from build123d import *

# Parameters (mm, degrees)
EXTRUDE_1_DEPTH      = 4
EXTRUDE_1_DEPTH_BACK = 0.4
SKETCH_1_R           = 4
SKETCH_1_3_R         = 4.175
SKETCH_1_3_R_2       = 4
CUT_EXTRUDE_1_DEPTH  = 3.6
CHAMFER_1_SIZE       = 0.2
FILLET_1_R           = 10


with BuildPart() as part:
    # 草图1 → 凸台-拉伸1 (new, two sides: drawn at the far end of the back side and taken through both)
    with BuildSketch(Plane.XY.offset(-EXTRUDE_1_DEPTH_BACK)):
        with BuildLine():
            ThreePointArc((5.196152423, 3), (-6, 0), (5.196152423, -3))
            Line((5.196152423, -3), (40.803847577, -3))
            ThreePointArc((40.803847577, -3), (52, 0), (40.803847577, 3))
            Line((40.803847577, 3), (5.196152423, 3))
        make_face()
        Circle(SKETCH_1_R, mode=Mode.SUBTRACT)
        with Locations((46, 0)):
            Circle(SKETCH_1_R, mode=Mode.SUBTRACT)
    extrude(amount=EXTRUDE_1_DEPTH + EXTRUDE_1_DEPTH_BACK)

    # 草图1<3> → 切除-拉伸1 (cut)
    # profile 1 of 2: a face of its own
    with BuildSketch(Plane.XY):
        Circle(SKETCH_1_3_R)
        Circle(SKETCH_1_3_R_2, mode=Mode.SUBTRACT)
    # profile 2 of 2: a face of its own
    with BuildSketch(Plane.XY):
        with Locations((46, 0)):
            Circle(SKETCH_1_3_R)
        with Locations((46, 0)):
            Circle(SKETCH_1_3_R_2, mode=Mode.SUBTRACT)
    extrude(amount=CUT_EXTRUDE_1_DEPTH, mode=Mode.SUBTRACT)

    # 倒角1
    # the kernel refuses this chamfer: 0.2 mm, written as the material it takes off along each edge
    with BuildSketch(Plane(origin=(0, 0, 3.6), x_dir=(1, 0, 0), z_dir=(0, -1, 0))) as chamfer_1_piece_1_section:
        Polygon((4, CHAMFER_1_SIZE), (4 + CHAMFER_1_SIZE, 0), (4, 0), align=None)
    chamfer_1_piece_1 = revolve(axis=Axis((0, 0, 3.6), (0, 0, 1)), mode=Mode.PRIVATE)
    chamfer_1_piece_1 = chamfer_1_piece_1 & Plane(origin=(0, 0, 3.709543273), x_dir=(1, 0, 0), z_dir=(0, 0, -1)) * Cylinder(4.175, 17, mode=Mode.PRIVATE)
    add(chamfer_1_piece_1, mode=Mode.SUBTRACT)
    with BuildSketch(Plane(origin=(46, 0, 3.6), x_dir=(1, 0, 0), z_dir=(0, -1, 0))) as chamfer_1_piece_2_section:
        Polygon((4, CHAMFER_1_SIZE), (4 + CHAMFER_1_SIZE, 0), (4, 0), align=None)
    chamfer_1_piece_2 = revolve(axis=Axis((46, 0, 3.6), (0, 0, 1)), mode=Mode.PRIVATE)
    chamfer_1_piece_2 = chamfer_1_piece_2 & Plane(origin=(46, 0, 3.709543273), x_dir=(1, 0, 0), z_dir=(0, 0, -1)) * Cylinder(4.175, 17, mode=Mode.PRIVATE)
    add(chamfer_1_piece_2, mode=Mode.SUBTRACT)
    with BuildSketch(Plane(origin=(46, 0, 0), x_dir=(1, 0, 0), z_dir=(0, -1, 0))) as chamfer_1_piece_3_section:
        Polygon((4, -CHAMFER_1_SIZE), (4 + CHAMFER_1_SIZE, 0), (4, 0), align=None)
    chamfer_1_piece_3 = revolve(axis=Axis((46, 0, 0), (0, 0, 1)), mode=Mode.PRIVATE)
    chamfer_1_piece_3 = chamfer_1_piece_3 & Plane(origin=(46, 0, -0.109543273), x_dir=(1, 0, 0), z_dir=(0, 0, -1)) * Cylinder(4.175, 17, mode=Mode.PRIVATE)
    add(chamfer_1_piece_3, mode=Mode.SUBTRACT)
    with BuildSketch(Plane(origin=(0, 0, 0), x_dir=(1, 0, 0), z_dir=(0, -1, 0))) as chamfer_1_piece_4_section:
        Polygon((4, -CHAMFER_1_SIZE), (4 + CHAMFER_1_SIZE, 0), (4, 0), align=None)
    chamfer_1_piece_4 = revolve(axis=Axis((0, 0, 0), (0, 0, 1)), mode=Mode.PRIVATE)
    chamfer_1_piece_4 = chamfer_1_piece_4 & Plane(origin=(0, 0, -0.109543273), x_dir=(1, 0, 0), z_dir=(0, 0, -1)) * Cylinder(4.175, 17, mode=Mode.PRIVATE)
    add(chamfer_1_piece_4, mode=Mode.SUBTRACT)

    # 圆角1
    fillet_1_edges = [part.edges().sort_by_distance(p)[0] for p in [
        (5.196152423, -3, 1.8),
        (5.196152423, 3, 1.8),
        (40.803847577, 3, 1.8),
        (40.803847577, -3, 1.8),
    ]]
    fillet(fillet_1_edges, radius=FILLET_1_R)


solid = part.part
Design review of the part built by this model. Coordinates are the model's own, in mm. A direction names the side the tool comes from. Coordinates: 2 decimals unless noted, no trailing zeros. Write each loop counter-clockwise with the first axis right and the second up, starting at its lowest first coordinate (ties: lowest second). Pieces come first, ordered by that corner, then holes. Notation, with made-up numbers: (9.25, -32) - (67.25, -32) arc R10 ccw to (67.25, -13) - close; hole circle Ø11 at (25.25, -33). An arc over 180 degrees is marked (long way). Use one line per item in the form item = value.
Q1. Insertion check: pin 1 Ø6.5 at (x, y) = (0, 0) entering from -Z; pin 2 Ø2 at (y, z) = (4.5, 2) entering from -X; pin 3 Ø1.3 at (x, z) = (17, 1.5) entering from +Y; pin 4 Ø1.5 at (y, z) = (-4, 1.5) entering from -X. Each pin has a flat end and moves straight along its axis. Give the tip position at first contact, or say it passes through.
Taken from the geometry:
pin_1 = through
pin_2 = -4.87
pin_3 = 3
pin_4 = -5.04
Q2. Consider section A-A (x = 46). Write out the cut boundary in (y, z) (3 decimals), plus the area to 3 significant figures.
Taken from the geometry:
outline = (-6, -0.4) - (-4, -0.4) - (-4, -0.2) - (-4.175, -0.025) - (-4.175, 3.625) - (-4, 3.8) - (-4, 4) - (-6, 4) - close; (4, -0.4) - (6, -0.4) - (6, 4) - (4, 4) - (4, 3.8) - (4.175, 3.625) - (4.175, -0.025) - (4, -0.2) - close
area = 16.3 mm^2
Q3. For probe 1 along X at (y, z) = (-2.75, 0.3); probe 2 along Y at (x, z) = (46, 1.6) (3 decimals); probe 3 along X at (y, z) = (-1.75, -0.2), list the stretches that pass through material, from the lowest coordinate up.
Taken from the geometry:
probe_1 = -5.33 to -3.14, 3.14 to 42.86, 49.14 to 51.33
probe_2 = -6 to -4.175, 4.175 to 6
probe_3 = -5.74 to -3.6, 3.6 to 42.4, 49.6 to 51.74
Q4. Consider section D-D (x = 29). Write out the cut boundary in (y, z), plus the area to 3 significant figures.
Taken from the geometry:
outline = (-3, -0.4) - (3, -0.4) - (3, 4) - (-3, 4) - close
area = 26.4 mm^2
Q5. Consider section B-B (y = 0). Write out the cut boundary in (x, z) (3 decimals), plus the area to 3 significant figures.
Taken from the geometry:
outline = (-6, -0.4) - (-4, -0.4) - (-4, -0.2) - (-4.175, -0.025) - (-4.175, 3.625) - (-4, 3.8) - (-4, 4) - (-6, 4) - close; (4, -0.4) - (42, -0.4) - (42, -0.2) - (41.825, -0.025) - (41.825, 3.625) - (42, 3.8) - (42, 4) - (4, 4) - (4, 3.8) - (4.175, 3.625) - (4.175, -0.025) - (4, -0.2) - close; (50, -0.4) - (52, -0.4) - (52, 4) - (50, 4) - (50, 3.8) - (50.175, 3.625) - (50.175, -0.025) - (50, -0.2) - close
area = 182 mm^2
Q6. Machinability: for faces 1 (the cylindrical face through (-6, 0, 2)), 2 (the cylindrical face through (6.2, 3.5, 1.8)), 3 (the cylindrical face through (39.693, -3.467, 1.831)), which of the approach directions +Z, -Z, +X, -X, +Y, -Y give a long, thin tool a straight path to every point of the face, cutting with its end or side? Answer none if there is none.
Taken from the geometry:
face_1 = +Z, -Z
face_2 = +Z, -Z, +Y
face_3 = +Z, -Z, -Y
Q7. Consider section C-C (z = 1.15). Write out the cut boundary in (x, y) (3 decimals).
Taken from the geometry:
outline = (3.498, -4.875) arc R10 cw to (9.327, -3) - (36.673, -3) arc R10 cw to (42.502, -4.875) arc R6 ccw (long way) to (42.502, 4.875) arc R10 cw to (36.673, 3) - (9.327, 3) arc R10 cw to (3.498, 4.875) arc R6 ccw (long way) to start; hole circle Ø8.35 at (0, 0); hole circle Ø8.35 at (46, 0)
